Verification items for the finished model (mm, model axes). Face numbers are marked on the shaded views. A direction names the side the tool comes from. Give positions to 0.01 mm unless a question says otherwise; leave off trailing zeros. Write each loop counter-clockwise with the first axis right and the second up, starting at its lowest first coordinate (ties: lowest second). Pieces come first, ordered by that corner, then holes. Notation, with made-up numbers: M 12.25,12.25 L 23.25,12.25 A10 cw 23.25,18.25 Z; hole C 68,-37 d5. An arc over 180 degrees is marked long. Answer as a JSON object with one key per item and string values.
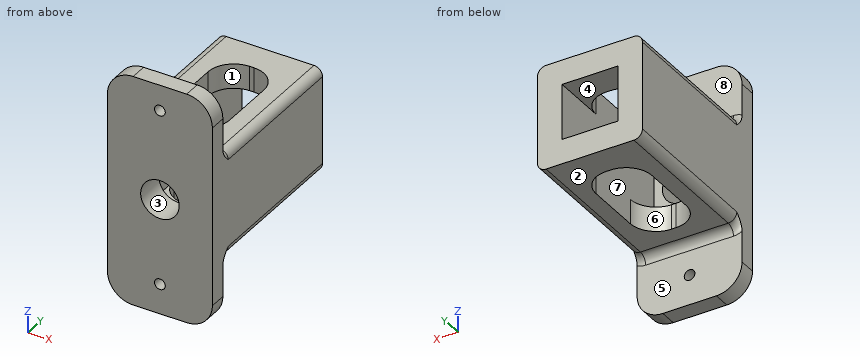
```python
from build123d import *

# Parameters (mm, degrees)
SKETCH_1_W          = 24.5
SKETCH_1_H          = 24.5
EXTRUDE_1_DEPTH     = 38
EXTRUDE_2_DEPTH     = 4
SKETCH_3_W          = 13
SKETCH_3_H          = 13
CUT_EXTRUDE_1_DEPTH = 35
SKETCH_4_R          = 4.5
CUT_EXTRUDE_2_DEPTH = 59.015622896
CUT_EXTRUDE_3_DEPTH = 60.873303734
FILLET_1_R          = 2
SKETCH_6_R          = 1.25
CUT_EXTRUDE_4_DEPTH = 63.488498942
FILLET_2_R          = 2


with BuildPart() as part:
    # Эскиз1 → Бобышка-Вытянуть1 (new body)
    with BuildSketch(Plane(origin=(0, 0, 0), x_dir=(1, 0, 0), z_dir=(0, 1, 0))):
        with Locations((12.25, 12.25)):
            Rectangle(SKETCH_1_W, SKETCH_1_H)
    extrude(amount=EXTRUDE_1_DEPTH)

    # Эскиз2 → Бобышка-Вытянуть2 (add)
    with BuildSketch(Plane.XZ):
        with BuildLine():
            Line((24.5, -24.5), (24.5, -33.25))
            ThreePointArc((24.5, -33.25), (22.742640687, -37.492640687), (18.5, -39.25))
            Line((18.5, -39.25), (6, -39.25))
            ThreePointArc((6, -39.25), (1.757359313, -37.492640687), (0, -33.25))
            Line((0, -33.25), (0, -24.5))
            Line((0, -24.5), (0, 0))
            Line((0, 0), (0, 8.75))
            ThreePointArc((0, 8.75), (1.757359313, 12.992640687), (6, 14.75))
            Line((6, 14.75), (18.5, 14.75))
            ThreePointArc((18.5, 14.75), (22.742640687, 12.992640687), (24.5, 8.75))
            Line((24.5, 8.75), (24.5, 0))
            Line((24.5, 0), (24.5, -24.5))
        make_face()
    extrude(amount=EXTRUDE_2_DEPTH)

    # Эскиз3 → Вырез-Вытянуть1 (cut)
    with BuildSketch(Plane(origin=(0, 38, 0), x_dir=(1, 0, 0), z_dir=(0, 1, 0))):
        with Locations((12.25, 12.25)):
            Rectangle(SKETCH_3_W, SKETCH_3_H)
    extrude(amount=-CUT_EXTRUDE_1_DEPTH, mode=Mode.SUBTRACT)

    # Эскиз4 → Вырез-Вытянуть2 (cut, through all)
    with BuildSketch(Plane(origin=(0, 3, 0), x_dir=(1, 0, 0), z_dir=(0, 1, 0))):
        with Locations(Location((12.25, 12.25, 0), (0, 0, 270))):
            Circle(SKETCH_4_R)
    extrude(amount=-CUT_EXTRUDE_2_DEPTH, mode=Mode.SUBTRACT)

    # Эскиз5 → Вырез-Вытянуть3 (cut, through all)
    with BuildSketch(Plane.XY):
        with BuildLine():
            Line((11.75, 31), (12.75, 31))
            ThreePointArc((12.75, 31), (16.992640687, 29.242640687), (18.75, 25))
            Line((18.75, 25), (18.75, 12))
            ThreePointArc((18.75, 12), (16.992640687, 7.757359313), (12.75, 6))
            Line((12.75, 6), (11.75, 6))
            ThreePointArc((11.75, 6), (7.507359313, 7.757359313), (5.75, 12))
            Line((5.75, 12), (5.75, 25))
            ThreePointArc((5.75, 25), (7.507359313, 29.242640687), (11.75, 31))
        make_face()
    extrude(amount=-CUT_EXTRUDE_3_DEPTH, mode=Mode.SUBTRACT)

    # Скругление1
    fillet_1_edges = [part.edges().sort_by_distance(p)[0] for p in [
        (0, 19, -24.5),
        (0, 19, 0),
        (24.5, 19, -24.5),
        (24.5, 19, 0),
    ]]
    fillet(fillet_1_edges, radius=FILLET_1_R)

    # Эскиз6 → Вырез-Вытянуть4 (cut, through all)
    with BuildSketch(Plane.XZ.offset(4)):
        with Locations(Location((12.25, 8.75, 0), (0, 0, 270))):
            Circle(SKETCH_6_R)
        with Locations(Location((12.25, -32.25, 0), (0, 0, 270))):
            Circle(SKETCH_6_R)
    extrude(amount=-CUT_EXTRUDE_4_DEPTH, mode=Mode.SUBTRACT)

    # Скругление2
    # the kernel refuses this fillet: 2 mm, written as the material it adds along each edge
    with BuildSketch(Plane(origin=(22.5, 0, -22.5), x_dir=(-0.8017442392976493, 0, 0.5976672776328263), z_dir=(-0.5976672776328263, 0, -0.8017442392976493))) as fillet_2_piece_1_section:
        with BuildLine():
            CenterArc((2 + FILLET_2_R, FILLET_2_R), FILLET_2_R, 180, 90)
            Line((2, FILLET_2_R), (2, 0))
            Line((2, 0), (2 + FILLET_2_R, 0))
        make_face()
    fillet_2_piece_1 = revolve(axis=Axis((22.5, 0, -22.5), (0, 1, 0)), revolution_arc=233.296989237, mode=Mode.PRIVATE)
    fillet_2_piece_1 = split(fillet_2_piece_1, bisect_by=Plane(origin=(24.5, 0.623256616, -23.99987789), z_dir=(-1, 0, 0)), keep=Keep.TOP, mode=Mode.PRIVATE)
    add(fillet_2_piece_1)
    with BuildSketch(Plane(origin=(2, 0, -22.5), x_dir=(0, 0, -1), z_dir=(1, 0, 0))) as fillet_2_piece_2_section:
        with BuildLine():
            CenterArc((2 + FILLET_2_R, FILLET_2_R), FILLET_2_R, 180, 90)
            Line((2, FILLET_2_R), (2, 0))
            Line((2, 0), (2 + FILLET_2_R, 0))
        make_face()
    fillet_2_piece_2 = revolve(axis=Axis((2, 0, -22.5), (0, 1, 0)), revolution_arc=233.296989237, mode=Mode.PRIVATE)
    fillet_2_piece_2 = split(fillet_2_piece_2, bisect_by=Plane(origin=(0, 0.334600406, -24.939550499), z_dir=(1, 0, 0)), keep=Keep.TOP, mode=Mode.PRIVATE)
    add(fillet_2_piece_2)
    with BuildSketch(Plane(origin=(2, 0, -2), x_dir=(0, 0, 1), z_dir=(1, 0, 0))) as fillet_2_piece_3_section:
        with BuildLine():
            CenterArc((2 + FILLET_2_R, -FILLET_2_R), FILLET_2_R, 90, 90)
            Line((2, -FILLET_2_R), (2, 0))
            Line((2, 0), (2 + FILLET_2_R, 0))
        make_face()
    fillet_2_piece_3 = revolve(axis=Axis((2, 0, -2), (0, -1, 0)), revolution_arc=233.296989237, mode=Mode.PRIVATE)
    fillet_2_piece_3 = split(fillet_2_piece_3, bisect_by=Plane(origin=(0, 0.334600403, 0.439550497), z_dir=(1, 0, 0)), keep=Keep.TOP, mode=Mode.PRIVATE)
    add(fillet_2_piece_3)
    with BuildSketch(Plane(origin=(22.5, 0, -2), x_dir=(-0.801744239297648, 0, -0.5976672776328278), z_dir=(-0.5976672776328278, 0, 0.801744239297648))) as fillet_2_piece_4_section:
        with BuildLine():
            CenterArc((2 + FILLET_2_R, -FILLET_2_R), FILLET_2_R, 90, 90)
            Line((2 + FILLET_2_R, 0), (2, 0))
            Line((2, 0), (2, -FILLET_2_R))
        make_face()
    fillet_2_piece_4 = revolve(axis=Axis((22.5, 0, -2), (0, -1, 0)), revolution_arc=233.296989237, mode=Mode.PRIVATE)
    fillet_2_piece_4 = split(fillet_2_piece_4, bisect_by=Plane(origin=(24.5, 0.623256909, -0.500122227), z_dir=(-1, 0, 0)), keep=Keep.TOP, mode=Mode.PRIVATE)
    add(fillet_2_piece_4)
    with BuildSketch(Plane(origin=(22.5, 0, -24.5), x_dir=(0, 0, -1), z_dir=(-1, 0, 0)), Plane(origin=(2, 0, 0), x_dir=(0, 0, 1), z_dir=(1, 0, 0))) as fillet_2_piece_5:
        with BuildLine():
            CenterArc((FILLET_2_R, -FILLET_2_R), FILLET_2_R, 90, 90)
            Line((0, -FILLET_2_R), (0, 0))
            Line((0, 0), (FILLET_2_R, 0))
        make_face()
    extrude(amount=20.5)


solid = part.part
```
1) Thickness scan on L1, parallel to Z at x = 9, y = 34.5; L2, parallel to X at y = -0.85, z = 8.75; L3, parallel to X at y = 11.5, z = -15. Record the ranges inside material, lowest first.
Completed:
{"L1": "z = -24.5 to -18.75, -5.75 to 0", "L2": "x = 0 to 11, 13.5 to 24.5", "L3": "x = 0 to 5.75, 18.75 to 24.5"}
2) Section check B-B on z = -12.25. Record the boundary of the cut face in (x, y), and give its area (3 significant figures).
Completed:
{"outline": "M 0,-4 L 7.75,-4 L 7.75,3 L 5.75,3 L 5.75,38 L 0,38 Z; M 16.75,-4 L 24.5,-4 L 24.5,38 L 18.75,38 L 18.75,3 L 16.75,3 Z", "area": "511 mm2"}
3) Section check D-D on z = -32.25. Record the boundary of the cut face in (x, y).
Completed:
{"outline": "M 0,-4 L 11,-4 L 11,0 L 0,0 Z; M 13.5,-4 L 24.5,-4 L 24.5,0 L 13.5,0 Z"}
4) Go/stop test with flat-tipped pins: pin 1 (6.5 mm diameter, centred on x = 11.5, y = 33.5, fed in from -Z); pin 2 (2 mm diameter, centred on y = 33.5, z = -24.5, fed in from -X); pin 3 (3 mm diameter, centred on x = 12.25, z = -32.25, fed in from +Y). Record where each tip stops, or that it passes through.
Completed:
{"pin 1": "stops at z = -24.5", "pin 2": "stops at x = 0.27", "pin 3": "stops at y = 0"}
5) Release check for a two-part mould opening along Z. For the marked faces 1, 2, 3 and 4 record: pulls with the +Z half, pulls with the -Z half, needs draft (parallel to the pull), parting line crosses it, or undercut.
Completed:
{"face 1": "needs draft", "face 2": "pulls with the -Z half", "face 3": "undercut", "face 4": "undercut"}
6) Section check C-C on x = 9. Record the boundary of the cut face in (y, z), and give its area (3 significant figures).
Completed:
{"outline": "M -4,-39.25 L 0,-39.25 L 0,-26.5 A2 cw 2,-24.5 L 6.67,-24.5 L 6.67,-18.75 L 3,-18.75 L 3,-15.36 L -4,-15.36 Z; M -4,-9.14 L 3,-9.14 L 3,-5.75 L 6.67,-5.75 L 6.67,0 L 2,0 A2 cw 0,2 L 0,14.75 L -4,14.75 Z; M 30.33,-24.5 L 38,-24.5 L 38,-18.75 L 30.33,-18.75 Z; M 30.33,-5.75 L 38,-5.75 L 38,0 L 30.33,0 Z", "area": "378 mm2"}
7) Access from +Z, -Z, +X, -X, +Y, -Y to the whole of each face (thin tool, end or side, straight path). Record for the marked faces 5, 6, 7 and 8.
Completed:
{"face 5": "-Z, +X, -X, +Y", "face 6": "+Z, -Z", "face 7": "none", "face 8": "+Z, +X, -X, +Y"}
8) Section check A-A on y = 19.5. Record the boundary of the cut face in (x, z).
Completed:
{"outline": "M 0,-22.5 A2 ccw 2,-24.5 L 5.75,-24.5 L 5.75,0 L 2,0 A2 ccw 0,-2 Z; M 18.75,-24.5 L 22.5,-24.5 A2 ccw 24.5,-22.5 L 24.5,-2 A2 ccw 22.5,0 L 18.75,0 Z"}
